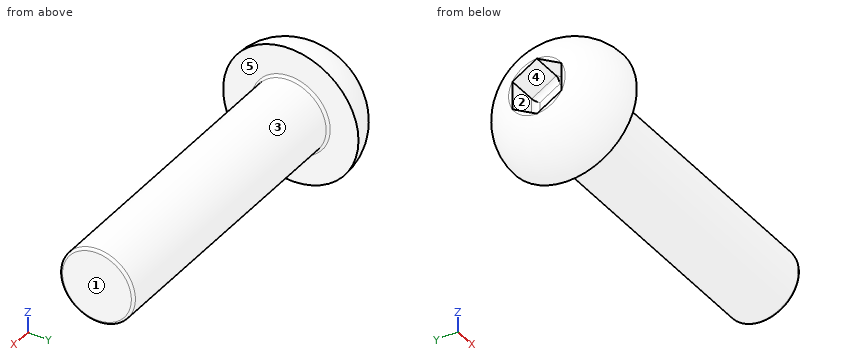
Autodesk Inventor part; units mm, degrees
ref_plane "YZ Plane" through (0, 0, 0) normal (1, 0, 0) x (0, 1, 0)
ref_plane "XZ Plane" through (0, 0, 0) normal (0, 1, 0) x (-1, 0, 0)
ref_plane "XY Plane" through (0, 0, 0) normal (0, 0, 1) x (1, 0, 0)
sketch "スケッチ1" plane through (0, 0, 0) normal (0, 0, 1) x (1, 0, 0)
  line L0 (0, 0) -> (12, 0)
  line L1 (12, 0) -> (12, 1.5)
  line L2 (12, 1.5) -> (0, 1.5)
  line L3 (0, 1.5) -> (0, 0)
  line L4 (0, 0) -> (0, 2.75)
  line L5 (0, 0) -> (-2, 0)
  line L6 (-2, 0) -> (0, 0)
  line L7 (-2, 0) -> (-2, 1.15)
  arc A0 (0, 2.75) -> (-2, 1.15) centre (-0.0403, 0.7504) ccw
  dimension "d0" = 1.5
  dimension "d1" = 12
  dimension "d3" = 2
  dimension "d4" = 2.75
  dimension "d5" = 1.15
  dimension "d6" = 2
revolve "回転1" add sketch "スケッチ1" angle 360 about axis through (-2, 0, 0) along (1, 0, 0)
thread "ねじ1"
sketch "スケッチ2" plane through (-2, 0, 0) normal (-1, 0, 0) x (0, 0, 1)
  circle A0 centre (0, 0) radius 1.15
  line L0 (-0.575, 0.9959) -> (0.575, 0.9959)
  line L1 (0.575, 0.9959) -> (1.15, 0)
  line L2 (1.15, 0) -> (0.575, -0.9959)
  line L3 (0.575, -0.9959) -> (-0.575, -0.9959)
  line L4 (-0.575, -0.9959) -> (-1.15, 0)
  line L5 (-1.15, 0) -> (-0.575, 0.9959)
  dimension "d10" = 1.15
  dimension "d11" = 1.9919
extrude "押し出し1" cut sketch "スケッチ2" against normal blind 1.4 contours L2 L3 L4 L5 L0 L1
fillet "フィレット1" radius 0.2 6 edges at (-0.6, 0.9959, 0) (-0.6, 0.498, 0.8625) (-0.6, 0.498, -0.8625) (-0.6, -0.498, -0.8625) (-0.6, -0.9959, 0) (-0.6, -0.498, 0.8625)
fillet "フィレット2" radius 0.1 1 edges at (0, -1.5, 0)
fillet "フィレット3" radius 0.1 1 edges at (12, -1.5, 0)
properties part number "ネジボタンM3L12" material "鋼"
Read the model definition and answer for the solid it produces. Units are mm, in the model's axes. Face numbers are marked on the shaded views. A direction names the side the tool comes from. Give positions to 0.01 mm unless a question says otherwise; leave off trailing zeros. Loops run counter-clockwise (first coordinate to the right, second up) from the corner with the lowest first, then second, coordinate; pieces in that order, holes last.
Item 1: The mould has two halves that part along Z. Classify the marked faces 3, 4 and 5: released by +Z, released by -Z, zero draft, split by the parting line, or undercut.
Item 2: Find the intervals of material crossed by line 1 along X through (y, z) = (1.85, -1.55); line 2 along X through (y, z) = (-0.7, 0.1); line 3 along Z through (x, y) = (9.5, 1.35), in increasing order.
Item 3: Each of these flat-tipped pins is pushed along its axis until it touches: pin 1 Ø0.9 at (x, z) = (-1.5, 0) entering from -Y; pin 2 Ø1 at (y, z) = (1.5, 2) entering from -X; pin 3 Ø3 at (x, z) = (10, 1.5) entering from +Y. Where does it stop, or does it pass through?
Item 4: The part is cut by section A-A (x = 9.75). Write down the section's boundary in (y, z), and give its area (3 significant figures).
Item 5: For the marked faces 1 and 2, determine the directions among +Z, -Z, +X, -X, +Y, -Y from which every point of the face is accessible in a straight line to the end or side of a thin tool.
Taken from the geometry:
1. face 3: split by the parting line
1. face 4: undercut
1. face 5: zero draft
2. line 1: x = -1.15 to 0
2. line 2: x = -0.6 to 12
2. line 3: z = -0.65 to 0.65
3. pin 1: stops at y = -2.48
3. pin 2: stops at x = -1.6
3. pin 3: stops at y = 1.5
4. outline: circle Ø3 at (0, 0)
4. area: 7.07 mm2
5. face 1: +Z, -Z, +X, +Y, -Y
5. face 2: -X
